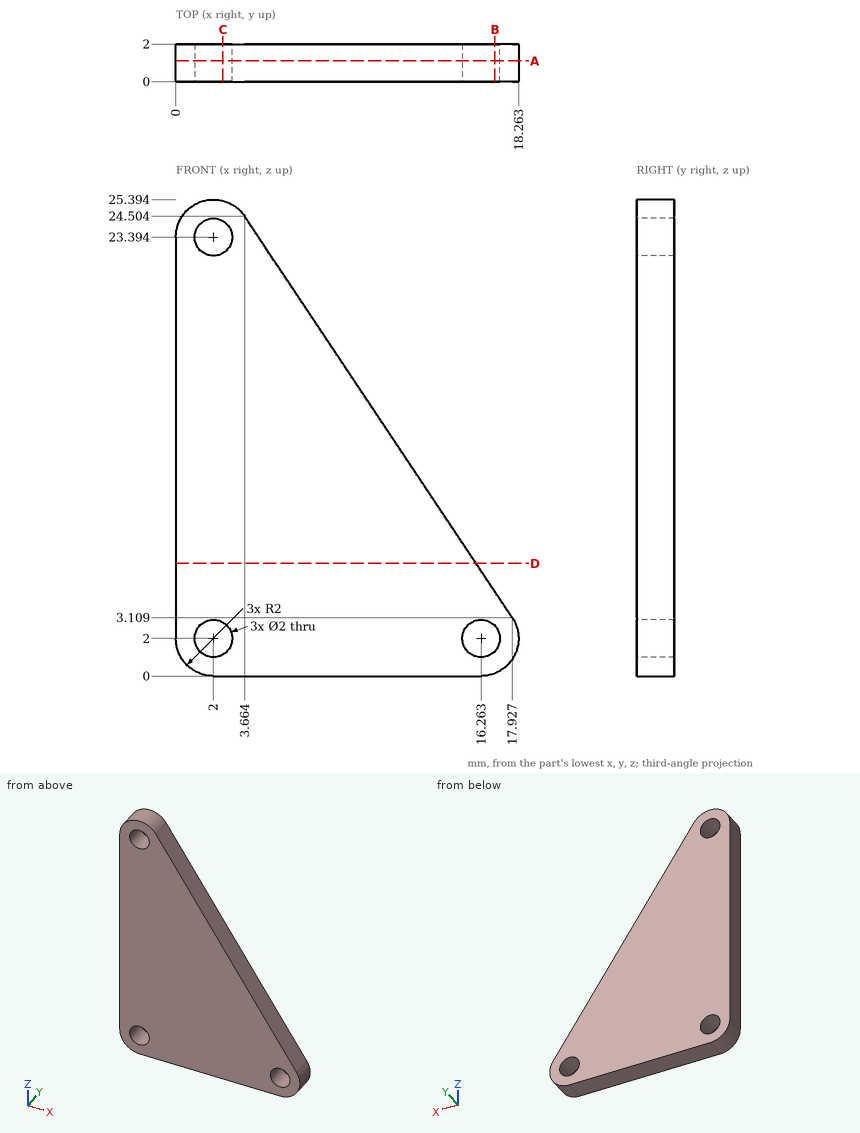
Input: dimensioned drawing with shaded views. Units: mm. Origin: part minimum x, y, z. Give positions to 0.01 mm unless a question says otherwise; leave off trailing zeros. Write each loop counter-clockwise with the first axis right and the second up, starting at its lowest first coordinate (ties: lowest second). Pieces come first, ordered by that corner, then holes. Notation, with made-up numbers: (45.25, 41) - (77.25, 41) arc R33 ccw to (77.25, 79) - close; hole circle Ø4 at (48, -21.5). An arc over 180 degrees is marked (long way). Write item = value, one per line. Start each with the question number.
1) Material intervals for L1, parallel to X at y = 0.9, z = 2; L2, parallel to Z at x = 1.75, y = 1.2 (1 decimal); L3, parallel to X at y = 0.2, z = 20.75 (1 decimal), sorted ascending. Write a range as [from, to].
2) Pin query (flat end, axial travel): pin 1 (1.8 mm diameter, centred on x = 16.263, z = 2, fed in from +Y). Return the tip coordinate at first contact, or that it passes through.
3) Cut plane B-B (x = 17). Return loops of the section in (y, z).
4) Cut plane A-A (y = 1.1). Return loops of the section in (x, z) (1 decimal).
5) Cut plane C-C (x = 2.5). Return loops of the section in (y, z).
6) Cut plane D-D (z = 6). Return loops of the section in (x, y).
Answers follow:
q1.L1 = [0, 1], [3, 15.26], [17.26, 18.26]
q1.L2 = [0, 1], [3, 22.4], [24.4, 25.4]
q1.L3 = [0, 6.2]
q2.pin_1 = through
q3.outline = (0, 0.14) - (2, 0.14) - (2, 1.32) - (0, 1.32) - close; (0, 2.68) - (2, 2.68) - (2, 4.5) - (0, 4.5) - close
q4.outline = (0, 2) arc R2 ccw to (2, 0) - (16.3, 0) arc R2 ccw to (17.9, 3.1) - (3.7, 24.5) arc R2 ccw to (0, 23.4) - close; hole circle Ø2 at (2, 2); hole circle Ø2 at (2, 23.4); hole circle Ø2 at (16.3, 2)
q5.outline = (0, 0) - (2, 0) - (2, 1.13) - (0, 1.13) - close; (0, 2.87) - (2, 2.87) - (2, 22.53) - (0, 22.53) - close; (0, 24.26) - (2, 24.26) - (2, 25.33) - (0, 25.33) - close
q6.outline = (0, 0) - (16, 0) - (16, 2) - (0, 2) - close
